Here's the drawing with two shaded views (mm, measured from the low corner). I have some questions. A direction names the side the tool comes from. Give positions to 0.01 mm unless a question says otherwise; leave off trailing zeros. Order: outer loops, then holes, each group sorted by start corner. A loop starts at its lowest first (then second) coordinate and runs counter-clockwise, first axis right, second up. Notation, with made-up numbers: (43, -38) - (82, -38) arc R26 ccw to (82, -6) - close; hole circle Ø6 at (3.5, -14). An arc over 180 degrees is marked (long way). Use one line per item in the form item = value. Start each with the question number.
1) Which directions (+Z, -Z, +X, -X, +Y, -Y) give clear straight access to the entire face, cutting with the end or side of a thin tool? Please do the marked faces 1 and 2.
2) We'd pull the mould along Z, two halves only. Please class the marked faces 3, 4 and 5: released by +Z, released by -Z, zero draft, split by the parting line, or undercut.
3) Suppose I cut it at A-A, the plane x = 12.5. Write out the boundary of the cut face in (y, z), and give its area (4 significant figures).
4) Please list where these lines run through material, in increasing order: probe 1 along Z at (x, y) = (15.75, 3.5); probe 2 along X at (y, z) = (15.25, 9.5).
5) Suppose I cut it at D-D, the plane z = 3.25. Write out the boundary of the cut face in (x, y).
6) For pin 1 (6 mm diameter, centred on y = 8, z = 13, fed in from -X); pin 2 (5 mm diameter, centred on x = 13, z = 8.5, fed in from +Y); pin 3 (5 mm diameter, centred on y = 12.5, z = 6, fed in from +X), each with a flat end and sliding along its axis, tell me the tip position at first contact or that it passes through.
7) Suppose I cut it at B-B, the plane y = 16.25. Write out the boundary of the cut face in (x, z).
8) Suppose I cut it at C-C, the plane z = 1. Write out the boundary of the cut face in (x, y), and give its area (3 significant figures).
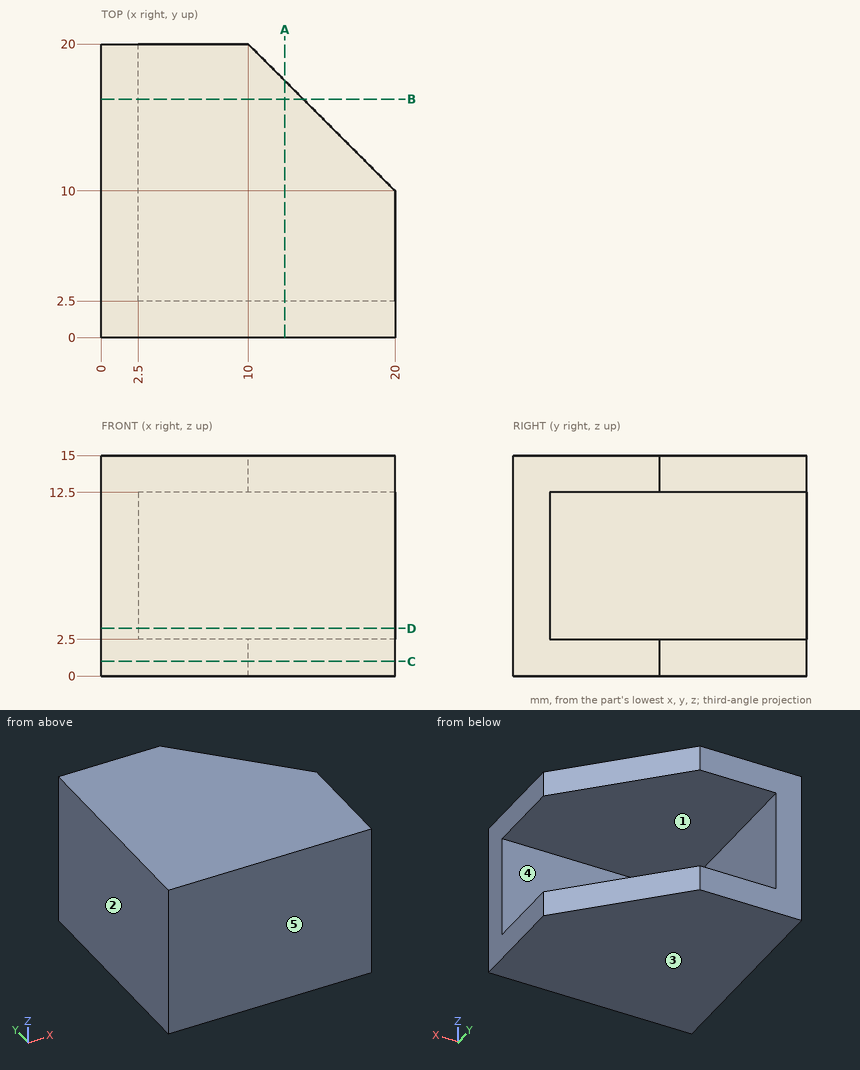
Result sheet:
q1.face_1 = +X, +Y
q1.face_2 = +Z, -Z, -X, +Y, -Y
q2.face_3 = released by -Z
q2.face_4 = undercut
q2.face_5 = zero draft
q3.outline = (0, 0) - (17.5, 0) - (17.5, 2.5) - (2.5, 2.5) - (2.5, 12.5) - (17.5, 12.5) - (17.5, 15) - (0, 15) - close
q3.area = 112.5 mm²
q4.probe_1 = 0 to 2.5, 12.5 to 15
q4.probe_2 = 0 to 2.5
q5.outline = (0, 0) - (20, 0) - (20, 2.5) - (2.5, 2.5) - (2.5, 20) - (0, 20) - close
q6.pin_1 = 0
q6.pin_2 = 2.5
q6.pin_3 = 2.5
q7.outline = (0, 0) - (13.75, 0) - (13.75, 2.5) - (2.5, 2.5) - (2.5, 12.5) - (13.75, 12.5) - (13.75, 15) - (0, 15) - close
q8.outline = (0, 0) - (20, 0) - (20, 10) - (10, 20) - (0, 20) - close
q8.area = 350 mm²
